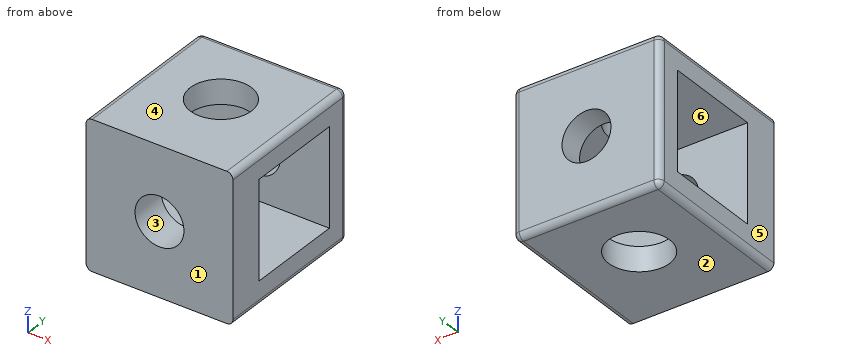
Autodesk Inventor part; units mm, degrees
ref_plane "YZ Plane" through (0, 0, 0) normal (1, 0, 0) x (0, 1, 0)
ref_plane "XZ Plane" through (0, 0, 0) normal (0, 1, 0) x (-1, 0, 0)
ref_plane "XY Plane" through (0, 0, 0) normal (0, 0, 1) x (1, 0, 0)
sketch "Sketch1" plane through (0, 0, 0) normal (0, 1, 0) x (-1, 0, 0)
  line L0 (6, -6) -> (-6, -6)
  line L1 (-6, -6) -> (-6, 6)
  line L2 (-6, 6) -> (6, 6)
  line L3 (6, 6) -> (6, -6)
  line L4 (6, -6) -> (-6, 6) construction
  line L5 (-6, -6) -> (6, 6) construction
  point P0 (0, 0)
  dimension "d0" = 12
  dimension "d1" = 12
extrude "Extrusion1" add sketch "Sketch1" along normal blind 13
sketch "Sketch2" plane through (6, 0, 6) normal (1, 0, 0) x (0, 0, -1)
  line L0 (0, 0) -> (0, 13)
  line L1 (0, 13) -> (12, 13)
  line L2 (12, 13) -> (12, 0)
  line L3 (12, 0) -> (0, 0)
  line L4 (10, 11) -> (2, 11)
  line L5 (2, 11) -> (2, 2)
  line L6 (2, 2) -> (10, 2)
  line L7 (10, 2) -> (10, 11)
  line L8 (2, 11) -> (10, 11)
  line L9 (10, 11) -> (10, 3)
  line L10 (10, 3) -> (2, 3)
  line L11 (2, 3) -> (2, 11)
  point P0 (6, 0)
  dimension "d4" = 2
  dimension "d5" = 8
  dimension "d6" = 8
extrude "Extrusion2" cut sketch "Sketch2" against normal blind 13 contours L7 L10 L5 L4
sketch "Sketch3" plane through (-6, 0, 6) normal (0, 0, 1) x (1, 0, 0)
  line L0 (12, 13) -> (12, 0)
  line L1 (12, 0) -> (0, 0)
  line L2 (0, 0) -> (0, 13)
  line L3 (0, 13) -> (12, 13)
  line L4 (0, 13) -> (12, 13)
  line L5 (12, 13) -> (12, 1)
  line L6 (12, 1) -> (0, 1)
  line L7 (0, 1) -> (0, 13)
  line L8 (12, 13) -> (0, 1) construction
  line L9 (0, 13) -> (12, 13) construction
  line L10 (0, 13) -> (12, 1) construction
  circle A0 centre (6, 7) radius 2.5
  point P0 (6, 0)
  dimension "d9" = 12
  dimension "d10" = 12
  dimension "d11" = 5
extrude "Extrusion3" cut sketch "Sketch3" against normal blind 13 contours A0
sketch "Sketch4" plane through (0, 13, 0) normal (0, 1, 0) x (1, 0, 0)
  circle A0 centre (0, 0) radius 2
  dimension "d14" = 4
extrude "Extrusion4" cut sketch "Sketch4" against normal blind 13
fillet "Fillet1" radius 0.5 8 edges at (0, 13, 6) (6, 6.5, 6) (-6, 6.5, 6) (-6, 6.5, -6) (6, 6.5, -6) (6, 13, 0) (0, 13, -6) (-6, 13, 0)
properties part number "Kutup Aki" material "Iron, Cast"
Work out the finished part from the listing and answer in its coordinate system (mm). Face numbers are marked on the shaded views. A direction names the side the tool comes from. Give positions to 0.01 mm unless a question says otherwise; leave off trailing zeros. Order: outer loops, then holes, each group sorted by start corner. A loop starts at its lowest first (then second) coordinate and runs counter-clockwise, first axis right, second up. Notation, with made-up numbers: (-2, 25.5) - (56, 25.5) arc R36 ccw to (56, 60.5) - close; hole circle Ø4 at (41.5, 33). An arc over 180 degrees is marked (long way). One line per item, written item: value. Start each with the question number.
1. Consider line 1 (Y direction, x = -0.5, z = 3.75); line 2 (Z direction, x = 0, y = 1.85); line 3 (Y direction, x = 0, z = -4.9). Determine where each line is inside the solid, lowest interval first.
2. Section D-D, the plane z = 3.25 is taken. Write down the section's boundary in (x, y).
3. Section A-A, the plane x = 0 is taken. Write down the section's boundary in (y, z).
4. For a pull along Z with two mould halves and no side action, classify the marked faces 1, 2, 3 and 4 as released by +Z, released by -Z, zero draft, split by the parting line, or undercut.
5. Section C-C, the plane y = 7 is taken. Write down the section's boundary in (x, z), then the cut area to 3 significant figures.
6. Which of the six approach directions +Z, -Z, +X, -X, +Y, -Y give full straight-line access (tool end or side, diameter ignored) to the marked faces 5 and 6?
7. Each of these flat-tipped pins is pushed along its axis until it touches: pin 1 Ø4 at (x, z) = (-2, -1) entering from -Y; pin 2 Ø2.5 at (x, z) = (0, 0) entering from -Y. Where does it stop, or does it pass through?
8. Section B-B, the plane z = 0 is taken. Write down the section's boundary in (x, y), then the cut area to 3 significant figures.
Filled sheet:
1. line 1: 0 to 3, 11 to 13
1. line 2: -6 to -2, 2 to 6
1. line 3: 0 to 4.5, 9.5 to 13
2. outline: (-6, 0) - (6, 0) - (6, 3) - (-6, 3) - close; (-6, 11) - (6, 11) - (6, 12.5) arc R0.5 ccw to (5.5, 13) - (-5.5, 13) arc R0.5 ccw to (-6, 12.5) - close
3. outline: (0, -6) - (4.5, -6) - (4.5, -4) - (3, -4) - (3, -2) - (0, -2) - close; (0, 2) - (3, 2) - (3, 4) - (4.5, 4) - (4.5, 6) - (0, 6) - close; (9.5, -6) - (12.5, -6) arc R0.5 ccw to (13, -5.5) - (13, -2) - (11, -2) - (11, -4) - (9.5, -4) - close; (9.5, 4) - (11, 4) - (11, 2) - (13, 2) - (13, 5.5) arc R0.5 ccw to (12.5, 6) - (9.5, 6) - close
4. face 1: zero draft
4. face 2: released by -Z
4. face 3: undercut
4. face 4: released by +Z
5. outline: (-6, -5.5) arc R0.5 ccw to (-5.5, -6) - (-2.5, -6) - (-2.5, -4) - (-6, -4) - close; (-6, 4) - (-2.5, 4) - (-2.5, 6) - (-5.5, 6) arc R0.5 ccw to (-6, 5.5) - close; (2.5, -6) - (5.5, -6) arc R0.5 ccw to (6, -5.5) - (6, -4) - (2.5, -4) - close; (2.5, 4) - (6, 4) - (6, 5.5) arc R0.5 ccw to (5.5, 6) - (2.5, 6) - close
5. area: 27.8 mm²
6. face 5: +Z, -Z, -X, +Y, -Y
6. face 6: +X, -X
7. pin 1: y = 0
7. pin 2: through
8. outline: (-6, 0) - (-2, 0) - (-2, 3) - (-6, 3) - close; (-6, 11) - (-2, 11) - (-2, 13) - (-5.5, 13) arc R0.5 ccw to (-6, 12.5) - close; (2, 0) - (6, 0) - (6, 3) - (2, 3) - close; (2, 11) - (6, 11) - (6, 12.5) arc R0.5 ccw to (5.5, 13) - (2, 13) - close
8. area: 39.9 mm²
